Autodesk Inventor part; units mm, degrees
ref_plane "YZ Plane" through (0, 0, 0) normal (1, 0, 0) x (0, 1, 0)
ref_plane "XZ Plane" through (0, 0, 0) normal (0, 1, 0) x (-1, 0, 0)
ref_plane "XY Plane" through (0, 0, 0) normal (0, 0, 1) x (1, 0, 0)
sketch "Sketch1" plane through (0, 0, 0) normal (1, 0, 0) x (0, 1, 0)
  line L0 (-15, 25) -> (15, 25)
  line L1 (15, 25) -> (15, -25)
  line L2 (15, -25) -> (-15, -25)
  line L3 (-15, -25) -> (-15, 25)
  line L4 (-15, 25) -> (15, -25) construction
  line L5 (15, 25) -> (-15, -25) construction
  point P0 (0, 0)
  dimension "d1" = 50
  dimension "d2" = 30
extrude "Extrusion1" add sketch "Sketch1" along normal blind 25
hole "Hole1" at (0, 0, 0) direction (1, 0, 0) diameter 10 depth 20
sketch "Sketch2" plane through (0, 15, 25) normal (0, 1, 0) x (1, 0, 0)
  line L0 (0, 25) -> (25, 25) construction
  line L1 (25, 50) -> (25, 0) construction
  line L2 (0, 50) -> (0, 0) construction
  point P0 (4, 25)
  point P1 (12, 25)
  dimension "d12" = 4
  dimension "d13" = 12
hole "Hole2" at (4, 15, 0) at (12, 15, 0) direction (0, -1, 0) diameter 3.242 end up to surface
sketch "Sketch3" plane through (25, 0, 0) normal (1, 0, 0) x (0, 0, -1)
  line L0 (-16.5, 0) -> (0, 0) construction
  line L1 (0, 0) -> (16.5, 0) construction
  dimension "d21" = 33
hole "Hole3" at (25, 0, 16.5) at (25, 0, -16.5) direction (-1, 0, 0) diameter 4.917 depth 17.1 tip angle 118
fillet "Fillet1" radius 2 4 edges at (12.5, 15, -25) (12.5, -15, -25) (12.5, -15, 25) (12.5, 15, 25)
properties part number "axle_tube_mount_10mm" material "Steel, Alloy"
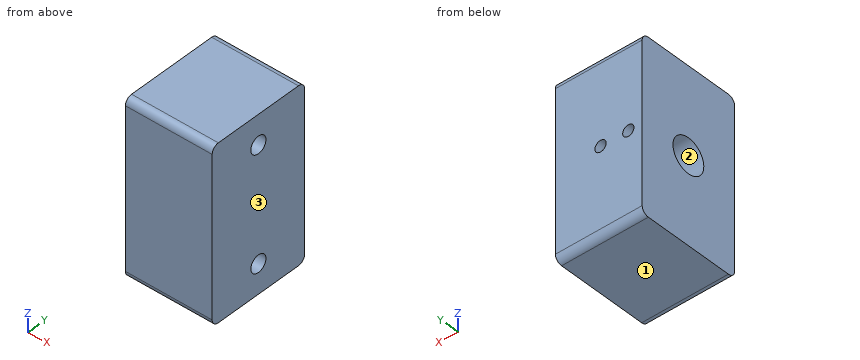
Work out the finished part from the listing and answer in its coordinate system (mm). Face numbers are marked on the shaded views. Give positions to 0.01 mm unless a question says otherwise; leave off trailing zeros. Write each loop counter-clockwise with the first axis right and the second up, starting at its lowest first coordinate (ties: lowest second). Pieces come first, ordered by that corner, then holes. Notation, with made-up numbers: (80.5, 28) - (92.5, 28) arc R28 ccw to (92.5, 59) - close; hole circle Ø3 at (63.25, 79.5). An arc over 180 degrees is marked (long way). Use one line per item in the form item = value.
1. Determine the mould class of the marked faces 1, 2 and 3 for opening direction Z: released by +Z, released by -Z, zero draft, split by the parting line, or undercut.
Filled in:
face_1 = released by -Z
face_2 = undercut
face_3 = zero draft
2. A cutting plane is placed at A-A (z = 0). Write down the section's boundary in (x, y).
Filled in:
outline = (0, -15) - (25, -15) - (25, 15) - (13.62, 15) - (13.62, 5) - (20, 5) - (20, -5) - (0, -5) - close; (0, 5) - (2.38, 5) - (2.38, 15) - (0, 15) - close; (5.62, 5) - (10.38, 5) - (10.38, 15) - (5.62, 15) - close
3. A cutting plane is placed at B-B (x = 14.25). Write down the section's boundary in (y, z), and give its area (3 significant figures).
Filled in:
outline = (-15, -23) arc R2 ccw to (-13, -25) - (13, -25) arc R2 ccw to (15, -23) - (15, 23) arc R2 ccw to (13, 25) - (-13, 25) arc R2 ccw to (-15, 23) - close; hole circle Ø10 at (0, 0); hole circle Ø4.92 at (0, -16.5); hole circle Ø4.92 at (0, 16.5)
area = 1,380 mm^2
4. Consider L1, parallel to Z at x = 13, y = 0; L2, parallel to Y at x = 21.25, z = 16.5; L3, parallel to Z at x = 21.25, y = -2. Determine where each line is inside the solid, lowest interval first.
Filled in:
L1 = -25 to -18.96, -14.04 to -5, 5 to 14.04, 18.96 to 25
L2 = -15 to -2.46, 2.46 to 15
L3 = -25 to -17.93, -15.07 to 15.07, 17.93 to 25
